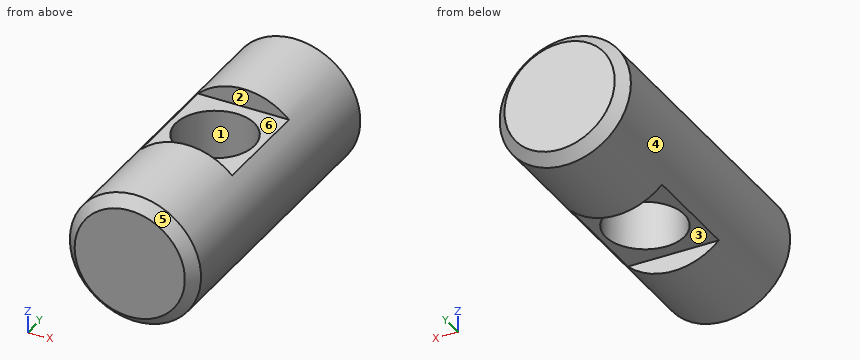
Autodesk Inventor part; units mm, degrees
ref_plane "YZ Plane" through (0, 0, 0) normal (1, 0, 0) x (0, 1, 0)
ref_plane "XZ Plane" through (0, 0, 0) normal (0, 1, 0) x (-1, 0, 0)
ref_plane "XY Plane" through (0, 0, 0) normal (0, 0, 1) x (1, 0, 0)
sketch "Sketch1" plane through (0, 0, 0) normal (0, 1, 0) x (-1, 0, 0)
  circle A0 centre (0, 0) radius 12.5
  dimension "d0" = 25
extrude "Extrusion1" add sketch "Sketch1" along normal blind 60
sketch "Sketch2" plane through (0, 0, 0) normal (0, 0, 1) x (1, 0, 0)
  line L0 (0, 0) -> (0, 30)
  circle A0 centre (0, 30) radius 7.5
  dimension "d3" = 30
  dimension "d4" = 15
extrude "Extrusion2" cut sketch "Sketch2" along normal mid plane 60
chamfer "Chamfer1" distance 2 angle 45 2 edges at (12.5, 60, 0) (12.5, 0, 0)
sketch "Sketch3" plane through (0, 0, 0) normal (1, 0, 0) x (0, 1, 0)
  line L0 (0, 0) -> (20, 0)
  line L1 (20, 0) -> (20, -9)
  line L2 (2, -12.5) -> (58, -12.5)
  line L3 (20, -9) -> (40, -9)
  line L4 (40, -9) -> (40, 9)
  line L5 (40, 9) -> (20, 9)
  line L6 (20, 9) -> (20, 0)
  line L7 (40, -9) -> (40, -15.8527)
  line L8 (40, -15.8527) -> (20, -15.8527)
  line L9 (20, -15.8527) -> (20, -9)
  line L10 (20, 9) -> (20, 19.7516)
  line L11 (20, 19.7516) -> (40, 19.7516)
  line L12 (40, 19.7516) -> (40, 9)
  dimension "d20" = 20
  dimension "d21" = 9
  dimension "d22" = 20
  dimension "d23" = 18
extrude "Extrusion3" cut sketch "Sketch3" along normal mid plane 25 contours L3 L7 L2 L9 | L10 L11 L12 L5 | L2 L7 L8 L9
properties part number "Pino Plataforma Deslizante"
Geometry check sheet. Reference: the model listing, model coordinates, mm. Face numbers are marked on the shaded views. A direction names the side the tool comes from. Round coordinates to 2 decimals unless told otherwise and drop trailing zeros. Loops run counter-clockwise (first coordinate to the right, second up) from the corner with the lowest first, then second, coordinate; pieces in that order, holes last. Notation, with made-up numbers: (11, 34) - (49, 34) arc R22 ccw to (49, 64) - close; hole circle Ø11 at (47.5, -9). An arc over 180 degrees is marked (long way). Use a Markdown table: item, result.
Q1. Access from +Z, -Z, +X, -X, +Y, -Y to the whole of each face (thin tool, end or side, straight path). Record for the marked faces 1, 2 and 3.
Solutions:
| item | result |
|---|---|
| face 1 | +Z, -Z |
| face 2 | +Z, +X, -X |
| face 3 | -Z, +X, -X |
Q2. Cross-section at C-C on z = 0. Record the cut outline in (x, y).
Solutions:
| item | result |
|---|---|
| outline | (-12.5, 2) - (-10.5, 0) - (10.5, 0) - (12.5, 2) - (12.5, 58) - (10.5, 60) - (-10.5, 60) - (-12.5, 58) - close; hole circle Ø15 at (0, 30) |
Q3. Cross-section at A-A on x = 0. Record the cut outline in (y, z), plus the area to 3 significant figures.
Solutions:
| item | result |
|---|---|
| outline | (0, -10.5) - (2, -12.5) - (20, -12.5) - (20, -9) - (22.5, -9) - (22.5, 9) - (20, 9) - (20, 12.5) - (2, 12.5) - (0, 10.5) - close; (37.5, -9) - (40, -9) - (40, -12.5) - (58, -12.5) - (60, -10.5) - (60, 10.5) - (58, 12.5) - (40, 12.5) - (40, 9) - (37.5, 9) - close |
| area | 1,080 mm2 |
Q4. Draft check along Y on the marked faces 4, 5 and 6. Enter one of: released by +Y, released by -Y, zero draft, split by the parting line, or undercut.
Solutions:
| item | result |
|---|---|
| face 4 | zero draft |
| face 5 | released by -Y |
| face 6 | undercut |
Q5. Cross-section at D-D on y = 15. Record the cut outline in (x, z).
Solutions:
| item | result |
|---|---|
| outline | circle Ø25 at (0, 0) |
Q6. Go/stop test with flat-tipped pins: P1, Ø2, axis at y = 12, z = 9, coming from the -X side; P2, Ø1.5, axis at y = 9.5, z = 6, coming from the +X side; P3, Ø12, axis at x = -8.5, y = 52.5, coming from the +Z side. Record where each tip stops, or that it passes through.
Solutions:
| item | result |
|---|---|
| P1 | stops at x = -9.6 |
| P2 | stops at x = 11.34 |
| P3 | stops at z = 12.25 |
Q7. Cross-section at B-B on y = 30. Record the cut outline in (x, z).
Solutions:
| item | result |
|---|---|
| outline | (-8.67, -9) - (-7.5, -9) - (-7.5, 9) - (-8.67, 9) arc R12.5 ccw to start; (7.5, -9) - (8.67, -9) arc R12.5 ccw to (8.67, 9) - (7.5, 9) - close |
Q8. Material ranges on line 1 (Y direction, x = 0, z = 3.25); line 2 (Z direction, x = -10, y = 9); line 3 (Z direction, x = -9, y = 38.5), recorded low to high.
Solutions:
| item | result |
|---|---|
| line 1 | y = 0 to 22.5, 37.5 to 60 |
| line 2 | z = -7.5 to 7.5 |
| line 3 | z = -8.67 to 8.67 |
